Design review of the part shown in the three views and the two pictorial views. Dimensions are in mm from the part's minimum x, y and z. A direction names the side the tool comes from. Coordinates: 2 decimals unless noted, no trailing zeros. Write each loop counter-clockwise with the first axis right and the second up, starting at its lowest first coordinate (ties: lowest second). Pieces come first, ordered by that corner, then holes. Notation, with made-up numbers: M 52.25,-3 L 76.25,-3 A30 cw 76.25,35 Z; hole C 46.5,5 d4. An arc over 180 degrees is marked long. Answer as a JSON object with one key per item and string values.
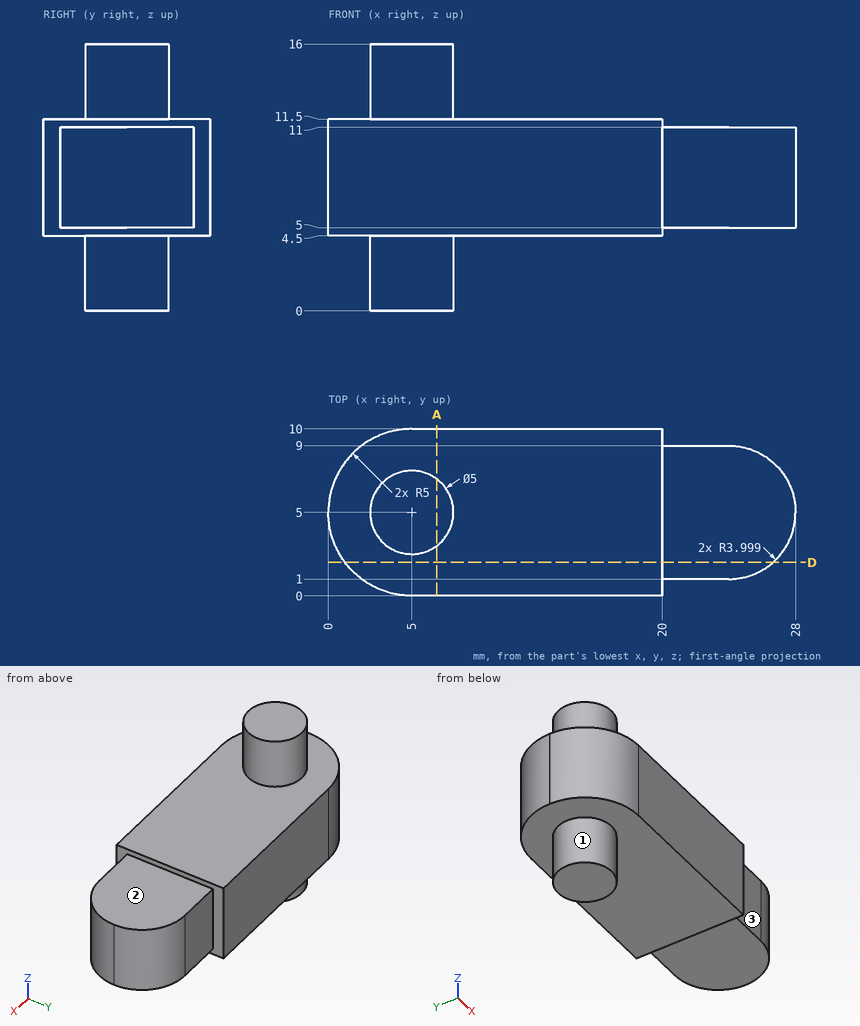
(1) For the marked faces 1, 2 and 3, list the 3-axis set-ups (+Z, -Z, +X, -X, +Y, -Y) from which the entire face can be reached by the end or side of a thin tool; tool diameter is ignored.
Results list:
{"face 1": "-Z", "face 2": "+Z, +X, +Y, -Y", "face 3": "+Z, -Z, +X, -Y"}
(2) Add section A-A on x = 6.5. Give the boundary of the cut face in (y, z), and give its area (3 significant figures).
Results list:
{"outline": "M 0,4.5 L 3,4.5 L 3,0 L 7,0 L 7,4.5 L 10,4.5 L 10,11.5 L 7,11.5 L 7,16 L 3,16 L 3,11.5 L 0,11.5 Z", "area": "106 mm²"}
(3) Add section D-D on y = 2. Give the boundary of the cut face in (x, z), and give its area (3 significant figures).
Results list:
{"outline": "M 1,4.5 L 20,4.5 L 20,5 L 26.65,5 L 26.65,11 L 20,11 L 20,11.5 L 1,11.5 Z", "area": "173 mm²"}
(4) For pin 1 Ø2 at (x, y) = (18.5, 7.5) entering from -Z; pin 2 Ø3 at (x, z) = (16.5, 2) entering from +Y; pin 3 Ø2.5 at (x, y) = (24, 3) entering from +Z; pin 4 Ø3 at (x, z) = (22, 7.5) entering from +Y, all flat-tipped, find the tip position at first contact; note any pin that passes through.
Results list:
{"pin 1": "z = 4.5", "pin 2": "through", "pin 3": "z = 11", "pin 4": "y = 9"}
(5) Wall thickness on line 1 along Z through (x, y) = (25, 2.5); line 2 along Z through (x, y) = (6.25, 9.25); line 3 along X through (y, z) = (0.5, 7) (1 decimal): over which ranges is each line inside the solid? List them lowest first. Write a range as from..to.
Results list:
{"line 1": "5..11", "line 2": "4.5..11.5", "line 3": "2.8..20"}
